from build123d import *

# Parameters (mm, degrees)
F0_W          = 5
F0_H          = 15
F1_DEPTH      = 2
F1_DEPTH_BACK = 2
F2_W          = 10
F2_H          = 5
F3_DEPTH      = 4
F6_R          = 2


with BuildPart() as f1:
    # F0 (on Front) → F1 (new body, two sides)
    with BuildSketch(Plane.XZ) as f1_sk:
        with Locations((0, 107.5)):
            Rectangle(F0_W, F0_H)
    extrude(amount=F1_DEPTH)
    extrude(f1_sk.sketch, amount=-F1_DEPTH_BACK)

    # F2 (on face) → F3 (join)
    with BuildSketch(Plane.XZ.offset(2)):
        with Locations((0, 110)):
            Rectangle(F2_W, F2_H)
    extrude(amount=-F3_DEPTH)

    # F4 (on Front) → F5 (revolve)
    with BuildSketch(Plane.XZ):
        with BuildLine():
            ThreePointArc((0, 101.582115), (-5.404094, 98.30643), (-5, 92))
            Line((-5, 92), (-20, 85))
            Line((-20, 85), (-8, 68))
            add(Edge.make_bspline(
                [(-8, 68), (-9.443204, 26.660192), (-10.776733, 21.775554), (-20, 10)],
                knots=[0, 0, 0, 0, 59.228372, 59.228372, 59.228372, 59.228372], degree=3))
            Line((-20, 10), (-20, 0))
            Line((-20, 0), (0, 0))
            Line((0, 0), (0, 101.582115))
        make_face()
    revolve(axis=Axis((0, 0, 50.791058), (0, 0, 1)))

    # F6
    f6_edges = [f1.edges().sort_by_distance(p)[0] for p in [
        (20, 0, 85),
    ]]
    fillet(f6_edges, radius=F6_R)


solid = f1.part
Here's how the part is built. I have some questions about the finished solid (model axes, mm). A direction names the side the tool comes from. Coordinates: 2 decimals unless noted, no trailing zeros. Order: outer loops, then holes, each group sorted by start corner. A loop starts at its lowest first (then second) coordinate and runs counter-clockwise, first axis right, second up. Notation, with made-up numbers: M -30.75,12 L 12.25,12 A24 ccw 12.25,44 Z; hole C 1,-1 d6. An arc over 180 degrees is marked long. Answer as CSV lines item,"result". Start each with the question number.
1. We'd pull the mould along Z, two halves only. Please class faces 4 (the flat face through (-5, 0, 110)), 5 (the flat face through (2.5, 0, 104)), 6 (the flat face through (-4, 0, 112.5)): released by +Z, released by -Z, zero draft, split by the parting line, or undercut.
2. I want a section at A-A, the plane z = 77.5. Write out the boundary of the cut face in (x, y).
3. For pin 1 (5 mm diameter, centred on x = 2, z = 84, fed in from -Y); pin 2 (0.8 mm diameter, centred on y = -1, z = 114, fed in from +X); pin 3 (10 mm diameter, centred on x = 12.5, z = 69.5, fed in from +Y), each with a flat end and sliding along its axis, tell me the tip position at first contact or that it passes through.
4. I need wall thicknesses on line 1 (Z direction, x = 11.5, y = -8); line 2 (Z direction, x = 16, y = -2); line 3 (Y direction, x = -6, z = 73). Which ranges of each line are inside material? Lowest first, please. Write a range as [from, to].
5. On a 3-axis mill with a long thin cutter (end or side, diameter ignored), from which of +Z, -Z, +X, -X, +Y, -Y can I reach the whole of each face in a straight line? I mean faces 1 (the flat face through (-2.5, 0, 114)), 2 (the flat face through (4, 0, 107.5)), 3 (the flat face through (5, 0, 110)). Say none if no direction works.
Recorded:
1,face 4,"zero draft"
1,face 5,"undercut"
1,face 6,"released by +Z"
2,outline,"C 0,0 d29.41"
3,pin 1,"stops at y = -18.99"
3,pin 2,"stops at x = 2.5"
3,pin 3,"stops at y = 7.3"
4,line 1,"z = [0, 19.06], [76.51, 87.8]"
4,line 2,"z = [0, 15.33], [79.51, 86.81]"
4,line 3,"y = [-9.85, 9.85]"
5,face 1,"+Z, -X, +Y, -Y"
5,face 2,"+X, +Y, -Y"
5,face 3,"+Z, +X, +Y, -Y"
